```python
from build123d import *

# Parameters (mm, degrees)
ESTRUSIONE_ESTRUSIONE1_DEPTH = 80
TAGLIO_ESTRUSIONE1_REACH     = 89.643


with BuildPart() as part:
    # Schizzo1 → Estrusione-Estrusione1 (new body)
    with BuildSketch(Plane(origin=(0, 0, 0), x_dir=(0, 0, -1), z_dir=(1, 0, 0))):
        Polygon((0, 35), (0, 30), (7.5, 30), (7.5, 5), (0, 5), (0, 0), (1, 0), (1, 4), (8.5, 4), (8.5, 31), (1, 31), (1, 35), align=None)
    extrude(amount=ESTRUSIONE_ESTRUSIONE1_DEPTH)

    # Schizzo2 → Taglio-Estrusione1 (cut, up to next)
    with BuildSketch(Plane.XY.offset(-7.5), mode=Mode.PRIVATE) as taglio_estrusione1_sk1:
        with BuildLine():
            Line((13.5, 20), (26.5, 20))
            ThreePointArc((26.5, 20), (29, 17.5), (26.5, 15))
            Line((26.5, 15), (13.5, 15))
            ThreePointArc((13.5, 15), (11, 17.5), (13.5, 20))
        make_face()
    taglio_estrusione1_tool1 = extrude(taglio_estrusione1_sk1.sketch, amount=-TAGLIO_ESTRUSIONE1_REACH, mode=Mode.PRIVATE) & part.part
    # Schizzo2 → Taglio-Estrusione1 (cut, up to next)
    with BuildSketch(Plane.XY.offset(-7.5), mode=Mode.PRIVATE) as taglio_estrusione1_sk2:
        with BuildLine():
            Line((53.5, 20), (66.5, 20))
            ThreePointArc((66.5, 20), (69, 17.5), (66.5, 15))
            Line((66.5, 15), (53.5, 15))
            ThreePointArc((53.5, 15), (51, 17.5), (53.5, 20))
        make_face()
    taglio_estrusione1_tool2 = extrude(taglio_estrusione1_sk2.sketch, amount=-TAGLIO_ESTRUSIONE1_REACH, mode=Mode.PRIVATE) & part.part
    add(taglio_estrusione1_tool1.solids().sort_by_distance((20, 17.5, -7.5))[0], mode=Mode.SUBTRACT)
    add(taglio_estrusione1_tool2.solids().sort_by_distance((60, 17.5, -7.5))[0], mode=Mode.SUBTRACT)


solid = part.part
```
The listing builds one solid part. Answer for the finished solid, in the listing's coordinates (mm). A direction names the side the tool comes from. Coordinates: 2 decimals unless noted, no trailing zeros. Loops run counter-clockwise (first coordinate to the right, second up) from the corner with the lowest first, then second, coordinate; pieces in that order, holes last. Notation, with made-up numbers: M 84,-23.5 L 113,-23.5 A12 cw 113,-18.5 Z; hole C 37,9 d3. An arc over 180 degrees is marked long. Answer as CSV lines item,"result". Start each with the question number.
(1) The mould has two halves that part along Y. Classify faces 4 (the flat face through (39, 2, -1)), 5 (the flat face through (39, 31, -5)), 6 (the cylindrical face through (29, 17.6, -8)): pulls with the +Y half, pulls with the -Y half, needs draft (parallel to the pull), parting line crosses it, or undercut.
(2) The part is cut by section C-C (x = 34.5). Give the vertices of the cut face in (y, z), and give its area (3 significant figures).
(3) The part is cut by section D-D (y = 25.5). Give the vertices of the cut face in (x, z), and give its area (3 significant figures).
(4) The part is cut by section B-B (z = -5.5). Give the vertices of the cut face in (x, y), and give its area (3 significant figures).
(5) Find the intervals of material crossed by L1, parallel to Y at x = 11.5, z = -5; L2, parallel to Y at x = 65, z = -8; L3, parallel to Z at x = 10, y = 21, in increasing order. Write a range as [from, to].
(6) For faces 1 (the flat face through (39, 18, -7.5)), 2 (the cylindrical face through (51, 17.4, -8)), 3 (the flat face through (39, 33, -1)), determine the directions among +Z, -Z, +X, -X, +Y, -Y from which every point of the face is accessible in a straight line to the end or side of a thin tool.
(7) The part is cut by section A-A (y = 17.5). Give the vertices of the cut face in (x, z), and give its area (3 significant figures).
(8) Given pin 1 (4 mm diameter, centred on x = 56.5, z = -6, fed in from +Y); pin 2 (12.5 mm diameter, centred on x = 29.5, y = 18.5, fed in from +Z); pin 3 (3 mm diameter, centred on x = 30, z = -6.5, fed in from -Y), each flat-ended and moving along its own axis, determine where each tip first touches the part or whether it passes through.
Determined:
1,face 4,"needs draft"
1,face 5,"pulls with the +Y half"
1,face 6,"undercut"
2,outline,"M 0,-1 L 4,-1 L 4,-8.5 L 31,-8.5 L 31,-1 L 35,-1 L 35,0 L 30,0 L 30,-7.5 L 5,-7.5 L 5,0 L 0,0 Z"
2,area,"50.0 mm2"
3,outline,"M 0,-8.5 L 80,-8.5 L 80,-7.5 L 0,-7.5 Z"
3,area,"80.0 mm2"
4,outline,"M 0,4 L 80,4 L 80,5 L 0,5 Z; M 0,30 L 80,30 L 80,31 L 0,31 Z"
4,area,"160 mm2"
5,L1,"[4, 5], [30, 31]"
5,L2,"[4, 15], [20, 31]"
5,L3,"[-8.5, -7.5]"
6,face 1,"+Z, +X, -X"
6,face 2,"+Z, -Z"
6,face 3,"-Z, +X, -X, +Y"
7,outline,"M 0,-8.5 L 11,-8.5 L 11,-7.5 L 0,-7.5 Z; M 29,-8.5 L 51,-8.5 L 51,-7.5 L 29,-7.5 Z; M 69,-8.5 L 80,-8.5 L 80,-7.5 L 69,-7.5 Z"
7,area,"44.0 mm2"
8,pin 1,"y = 31"
8,pin 2,"z = -7.5"
8,pin 3,"y = 4"
